CAD build for the part. Positions are in the model's coordinates, mm. Face numbers are marked on the shaded views. A direction names the side the tool comes from. Give positions to 0.01 mm unless a question says otherwise; leave off trailing zeros. Write each loop counter-clockwise with the first axis right and the second up, starting at its lowest first coordinate (ties: lowest second). Pieces come first, ordered by that corner, then holes. Notation, with made-up numbers: (87.5, -38) -> (132.5, -38) arc R27 cw to (132.5, -20) -> close; hole circle Ø2 at (42.25, 77.25). An arc over 180 degrees is marked (long way). Answer in a Markdown table with one row per item. Add a question column.
```python
from build123d import *

# Parameters (mm, degrees)
F0_W     = 41
F0_H     = 90
F1_DEPTH = 34
F2_W     = 35
F2_H     = 29
F3_DEPTH = 86
F4_W     = 5.5
F4_H     = 5.5
F4_R     = 3.75
F4_H_2   = 3
F4_R_2   = 1.5
F5_DEPTH = 4
F6_W     = 5
F6_H     = 2.5
F6_W_2   = 3
F6_H_2   = 5
F7_DEPTH = 2.5
F8_W     = 5
F8_H     = 27
F9_DEPTH = 4


with BuildPart() as f1:
    # F0 (on Top) → F1 (new body)
    with BuildSketch(Plane.XY):
        with Locations((-1.702341, 4.193077)):
            Rectangle(F0_W, F0_H)
    extrude(amount=F1_DEPTH)

    # F2 (on face) → F3 (cut)
    with BuildSketch(Plane.XZ.offset(40.806923)):
        with Locations((-1.702341, 17)):
            Rectangle(F2_W, F2_H)
    extrude(amount=-F3_DEPTH, mode=Mode.SUBTRACT)

    # F4 (on face) → F5 (cut, through all)
    with BuildSketch(Plane(origin=(0, 49.193077, 0), x_dir=(-1, 0, 0), z_dir=(0, 1, 0))):
        with Locations((-8.047659, 7.522329)):
            Rectangle(F4_W, F4_H)
        with Locations((1.702341, 17)):
            Circle(F4_R)
        with Locations((10.567795, 28.5)):
            Rectangle(F4_W, F4_H_2)
        with Locations((10.202341, 17)):
            Circle(F4_R_2)
        with Locations((-6.797659, 17)):
            Circle(F4_R_2)
    extrude(amount=-F5_DEPTH, mode=Mode.SUBTRACT)

    # F6 (on face) → F7 (join)
    with BuildSketch(Plane.XZ.offset(40.806923)):
        with Locations((-1.702341, 32.75)):
            Rectangle(F6_W, F6_H)
        with Locations((-20.702341, 17)):
            Rectangle(F6_W_2, F6_H_2)
        with Locations((17.297659, 17)):
            Rectangle(F6_W_2, F6_H_2)
        with Locations((-1.702341, 1.25)):
            Rectangle(F6_W, F6_H)
    extrude(amount=F7_DEPTH)

    # F8 (on face) → F9 (join)
    with BuildSketch(Plane(origin=(0, 0, 0), x_dir=(1, 0, 0), z_dir=(0, 0, -1))):
        with Locations((-19.702341, -9.693077)):
            Rectangle(F8_W, F8_H)
        with Locations((16.297659, -9.693077)):
            Rectangle(F8_W, F8_H)
    extrude(amount=F9_DEPTH)


solid = f1.part
```
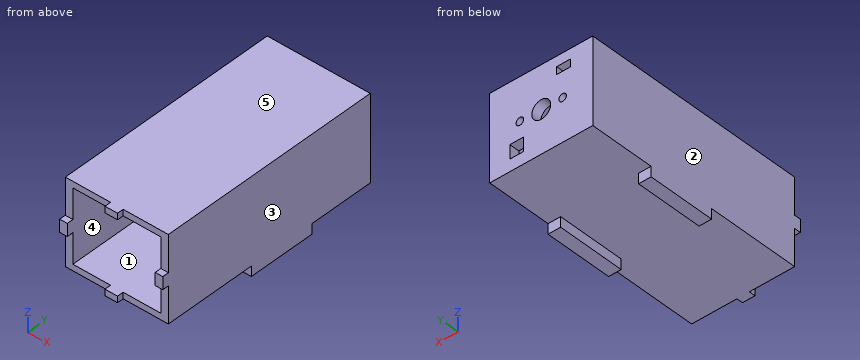
Item 1: Drop flat-ended pins along their axis: pin 1 Ø1.2 at (x, z) = (16.5, -2.5) entering from +Y; pin 2 Ø1.2 at (x, y) = (8.5, 47) entering from -Z; pin 3 Ø16 at (x, z) = (12, 3.5) entering from -Y. Give the stop position or say it passes through.
Item 2: Slice it at B-B, the plane z = 17. List the corners of the cut face in (x, y), then the cut area to 3 significant figures.
Item 3: Mould opens along Z. For the marked faces 3, 4 and 5 say: released by +Z, released by -Z, zero draft, split by the parting line, or undercut.
Item 4: Probe L1, parallel to X at y = 16, z = 22; L2, parallel to Z at x = -9.5, y = 40; L3, parallel to Y at x = -15, z = 23. List the from-to ranges inside material, lowest first. Write a range as from..to.
Item 5: Slice it at A-A, the plane y = 20. List the corners of the cut face in (x, z), then the cut area to 3 significant figures.
Item 6: Slice it at D-D, the plane y = 33. List the corners of the cut face in (x, z), then the cut area to 3 significant figures.
Item 7: Which spindle directions (+Z, -Z, +X, -X, +Y, -Y) get a long thin tool onto all of the face, cutting with end or side? Do the marked faces 1 and 2. Say none if no direction does.
Item 8: Slice it at C-C, the plane x = -2. List the corners of the cut face in (y, z), then the cut area to 3 significant figures.
Answer key:
| question | item | result |
|---|---|---|
| 1 | pin 1 | stops at y = 23.19 |
| 1 | pin 2 | stops at z = 0 |
| 1 | pin 3 | stops at y = -40.81 |
| 2 | outline | (-22.2, -43.31) -> (-19.2, -43.31) -> (-19.2, 45.19) -> (-11.7, 45.19) -> (-11.7, 49.19) -> (-22.2, 49.19) -> close; (-8.7, 45.19) -> (-5.45, 45.19) -> (-5.45, 49.19) -> (-8.7, 49.19) -> close; (2.05, 45.19) -> (5.3, 45.19) -> (5.3, 49.19) -> (2.05, 49.19) -> close; (8.3, 45.19) -> (15.8, 45.19) -> (15.8, -43.31) -> (18.8, -43.31) -> (18.8, 49.19) -> (8.3, 49.19) -> close |
| 2 | area | 641 mm² |
| 3 | face 3 | zero draft |
| 3 | face 4 | undercut |
| 3 | face 5 | released by +Z |
| 4 | L1 | x = -22.2..-19.2, 15.8..18.8 |
| 4 | L2 | z = 0..2.5, 31.5..34 |
| 4 | L3 | y = 45.19..49.19 |
| 5 | outline | (-22.2, -4) -> (-17.2, -4) -> (-17.2, 0) -> (13.8, 0) -> (13.8, -4) -> (18.8, -4) -> (18.8, 34) -> (-22.2, 34) -> close; hole (-19.2, 2.5) -> (15.8, 2.5) -> (15.8, 31.5) -> (-19.2, 31.5) -> close |
| 5 | area | 419 mm² |
| 6 | outline | (-22.2, 0) -> (18.8, 0) -> (18.8, 34) -> (-22.2, 34) -> close; hole (-19.2, 2.5) -> (15.8, 2.5) -> (15.8, 31.5) -> (-19.2, 31.5) -> close |
| 6 | area | 379 mm² |
| 7 | face 1 | -Y |
| 7 | face 2 | +Z, -Z, -X, +Y, -Y |
| 8 | outline | (-43.31, 0) -> (49.19, 0) -> (49.19, 13.26) -> (45.19, 13.26) -> (45.19, 2.5) -> (-43.31, 2.5) -> close; (-43.31, 31.5) -> (45.19, 31.5) -> (45.19, 20.74) -> (49.19, 20.74) -> (49.19, 34) -> (-43.31, 34) -> close |
| 8 | area | 549 mm² |
